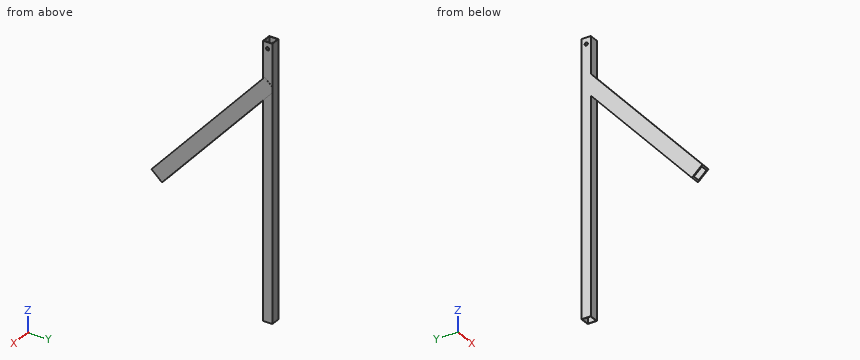
from build123d import *

# Parameters (mm, degrees)
SKETCH2_W           = 26.352182783
SKETCH2_H           = 26.352182783
SKETCH2_W_2         = 23.8
SKETCH2_H_2         = 23.8
BOSS_EXTRUDE1_DEPTH = 385
SKETCH3_R           = 4.5
CUT_EXTRUDE1_DEPTH  = 387.799528276
SKETCH4_W           = 26.521697909
SKETCH4_H           = 40
SKETCH4_W_2         = 19.891273431
SKETCH4_H_2         = 30
BOSS_EXTRUDE2_DEPTH = 480
CUT_EXTRUDE2_DEPTH  = 500.249823585


with BuildPart() as part:
    # Sketch2 → Boss-Extrude1 (new, symmetric)
    with BuildSketch(Plane.XY):
        with Locations((-13.176091391, 13.176091391)):
            Rectangle(SKETCH2_W, SKETCH2_H)
        with Locations((-13.091333829, 13.176091663)):
            Rectangle(SKETCH2_W_2, SKETCH2_H_2, mode=Mode.SUBTRACT)
    extrude(amount=BOSS_EXTRUDE1_DEPTH, both=True)

    # Sketch3 → Cut-Extrude1 (cut, through all)
    with BuildSketch(Plane.ZY.offset(26.352182783)):
        with Locations((367, 13)):
            Circle(SKETCH3_R)
    extrude(amount=-CUT_EXTRUDE1_DEPTH, mode=Mode.SUBTRACT)

    # Sketch4 → Boss-Extrude2 (add)
    with BuildSketch(Plane(origin=(0, -176.990909821, -196.568319459), x_dir=(1, 0, 0), z_dir=(0, 0.6691306063588407, 0.7431448254774101))):
        with Locations((-13.091333828, -168.046187829)):
            Rectangle(SKETCH4_W, SKETCH4_H)
        with Locations((-13.091333829, -168.046187829)):
            Rectangle(SKETCH4_W_2, SKETCH4_H_2, mode=Mode.SUBTRACT)
    extrude(amount=BOSS_EXTRUDE2_DEPTH)

    # Sketch5 → Cut-Extrude2 (cut, through all)
    with BuildSketch(Plane.ZY.offset(26.352182783)):
        Polygon((266.244447792, 26.352182783), (250.51862, 26.352182783), (259.203432202, 34.172022814), align=None)
    extrude(amount=-CUT_EXTRUDE2_DEPTH, mode=Mode.SUBTRACT)


solid = part.part
Could you check a few things on this model? Use its own coordinates, in mm. Give positions to 0.01 mm unless a question says otherwise; leave off trailing zeros. Order: outer loops, then holes, each group sorted by start corner. A loop starts at its lowest first (then second) coordinate and runs counter-clockwise, first axis right, second up. Notation, with made-up numbers: (10, -11.75) - (52, -11.75) arc R22 cw to (52, 14.25) - close; hole circle Ø5 at (9, 52.5). An arc over 180 degrees is marked (long way). Return JSON: item names as keys, results as strings. Group by question number.
Q1. Suppose I cut it at B-B, the plane z = 77. Please give me the cut outline in (x, y).
Q2. Suppose I cut it at D-D, the plane x = -17.25. Please give me the cut outline in (y, z), and give its area (3 significant figures).
Q3. Will these pins go through, and if not, where does the flat tip stop? pin 1 Ø8 at (x, z) = (-14.5, 94.5) entering from -Y; pin 2 Ø13 at (x, z) = (-19.5, 311.5) entering from -Y; pin 3 Ø13 at (x, z) = (-11, -55.5) entering from -Y; pin 4 Ø5.5 at (y, z) = (13, 367) entering from +X.
Q4. Suppose I cut it at A-A, the plane z = -327.5. Please give me the cut outline in (x, y).
Q5. Please list where these lines run through material, in increasing order: line 1 along Y through (x, z) = (-17, -167); line 2 along Y through (x, z) = (-9, -18); line 3 along Y through (x, z) = (-8, -40). Write a range as [from, to].
Q6. Suppose I cut it at C-C, the plane y = -109. Please give me the cut outline in (x, z).
Resolved:
{
 "1": {"outline": "(-26.35, -183.71) - (0.17, -183.71) - (0.17, -129.88) - (-26.35, -129.88) - close; (-26.35, 0) - (0, 0) - (0, 26.35) - (-26.35, 26.35) - close; hole (-24.99, 1.28) - (-1.19, 1.28) - (-1.19, 25.08) - (-24.99, 25.08) - close; hole (-23.04, -176.98) - (-3.15, -176.98) - (-3.15, -136.61) - (-23.04, -136.61) - close"},
 "2": {"outline": "(-316.74, -70.74) - (-313.02, -74.09) - (0, 273.56) - (0, 228.72) - (-290.73, -94.16) - (-287.01, -97.51) - (0, 221.25) - (0, -385) - (1.28, -385) - (1.28, 222.67) - (25.08, 249.1) - (25.08, -385) - (26.35, -385) - (26.35, 385) - (25.08, 385) - (25.08, 256.57) - (1.28, 230.14) - (1.28, 274.98) - (8.16, 282.62) - (4.45, 285.97) - (1.28, 282.45) - (1.28, 385) - (0, 385) - (0, 281.03) - close", "area": "6,690 mm2"},
 "3": {"pin 1": "stops at y = -171.55", "pin 2": "stops at y = 0", "pin 3": "stops at y = -308.87", "pin 4": "passes through"},
 "4": {"outline": "(-26.35, 0) - (0, 0) - (0, 26.35) - (-26.35, 26.35) - close; hole (-24.99, 1.28) - (-1.19, 1.28) - (-1.19, 25.08) - (-24.99, 25.08) - close"},
 "5": {"line 1": "y = [0, 1.28], [25.08, 26.35]", "line 2": "y = [-269.25, -262.52], [-222.15, -215.42], [0, 1.28], [25.08, 26.35]", "line 3": "y = [-289.06, -282.33], [-241.96, -235.23], [0, 1.28], [25.08, 26.35]"},
 "6": {"outline": "(-26.35, 100.19) - (0.17, 100.19) - (0.17, 159.97) - (-26.35, 159.97) - close; hole (-23.04, 107.67) - (-3.15, 107.67) - (-3.15, 152.5) - (-23.04, 152.5) - close"}
}
